Part model, mm, in its own coordinate system. A direction names the side the tool comes from. Give positions to 0.01 mm unless a question says otherwise; leave off trailing zeros. Write each loop counter-clockwise with the first axis right and the second up, starting at its lowest first coordinate (ties: lowest second). Pieces come first, ordered by that corner, then holes. Notation, with made-up numbers: (4.5, 77) - (18.5, 77) arc R26 cw to (18.5, 103) - close; hole circle Ø6 at (61, 10). An arc over 180 degrees is marked (long way). Answer in a Markdown table with one row per item. Add a question column.
1. Band-saw the part on B-B on y = -3. Write the cut outline in (x, z), plus the area to 3 significant figures.
2. Drop flat-ended pins along their axis: pin 1 Ø1.5 at (x, z) = (11, -72) entering from -Y; pin 2 Ø4.5 at (x, z) = (1, -8) entering from +Y; pin 3 Ø12 at (y, z) = (9, -81.5) entering from +X. Give the stop position or say it passes through.
3. Probe line 1 along Z through (x, y) = (8, -3.5); line 2 along Z through (x, y) = (-10, -13); line 3 along Y through (x, z) = (-1, -3). List the from-to ranges inside material, lowest first.
4. Band-saw the part on D-D on y = -10. Write the cut outline in (x, z), plus the area to 3 significant figures.
5. Which spindle directions (+Z, -Z, +X, -X, +Y, -Y) get a long thin tool onto all of the face, cutting with end or side? Do faces 1 (the flat face through (4.03, -2.29, 12.08)), 2 (the flat face through (1, 5, -31.75)), 3 (the flat face through (-4.03, 2.29, 12.08)). Say none if no direction does.
Autodesk Inventor part; units mm, degrees
ref_plane "YZ Plane" through (0, 0, 0) normal (1, 0, 0) x (0, 1, 0)
ref_plane "XZ Plane" through (0, 0, 0) normal (0, 1, 0) x (-1, 0, 0)
ref_plane "XY Plane" through (0, 0, 0) normal (0, 0, 1) x (1, 0, 0)
sketch "Sketch1" plane through (0, 0, 0) normal (0, 0, 1) x (1, 0, 0)
  line L0 (5.4993, 0) -> (2.7496, -4.7625)
  line L1 (2.7496, -4.7625) -> (-2.7496, -4.7625)
  line L2 (-2.7496, -4.7625) -> (-5.4993, 0)
  line L3 (-5.4993, 0) -> (-2.7496, 4.7625)
  line L4 (-2.7496, 4.7625) -> (2.7496, 4.7625)
  line L5 (2.7496, 4.7625) -> (5.4993, 0)
  circle A0 centre (0, 0) radius 0.0127
  dimension "d0" = 9.525
  dimension "d6" = 0.0254
extrude "Extrusion2" add sketch "Sketch1" along normal mid plane 114.3
sketch "Sketch4" plane through (0, 0, -57.15) normal (0, 0, -1) x (-1, 0, 0)
  circle A0 centre (0, 0) radius 0.0127
  circle A1 centre (0, 0) radius 12.7
  dimension "d10" = 25.4
extrude "Extrusion4" add sketch "Sketch4" against normal blind 19.05
thicken "Reduce Hex Shaft" operation add thickness 0.127 both sides no extend neighbours yes toward (0, -1, 0) faces at (0.9165, 4.7625, -6.35) (4.5827, 1.5875, -6.35) (3.6662, -3.175, -6.35) (-3.6662, 3.175, -6.35) (-4.5827, -1.5875, -6.35) (-0.9165, -4.7625, -6.35)
sketch "Sketch5" plane through (0, 0, -38.1) normal (0, 0, 1) x (1, 0, 0)
  circle A0 centre (0, 0) radius 6.35
  dimension "d15" = 12.7
extrude "Extrusion5" add sketch "Sketch5" along normal blind 6.35
thicken "Reduce Base Bushing" operation add thickness 0.127 both sides no extend neighbours yes toward (-0.9967573, 0.0804666, 0) faces at (6.3294, -0.511, -33.8667)
sketch "Sketch8" plane through (0, 0, -57.15) normal (0, 0, -1) x (-1, 0, 0)
  circle A0 centre (0, 0) radius 19.05
  dimension "d28" = 38.1
extrude "Extrusion7" add sketch "Sketch8" along normal blind 50.8
equation "\"d0\" = hexSize"
equation "\"d4\" = length"
equation "\"d13\" = printOffset"
equation "\"d14\" = printOffset"
equation "\"d15\" = bushingForBaseHole"
equation "\"d16\" = sideOfBase"
equation "\"d20\" = printOffset"
equation "\"d21\" = printOffset"
equation "\"hexSize\" = 9.525"
equation "\"length\" = 114.3"
equation "\"printOffset\" = 0.127"
equation "\"bushingForBaseHole\" = 12.7"
equation "\"sideOfBase\" = 6.35"
properties part number "3_8x6_5-inchHexShaft" material "PC/ABS Plastic"
Values:
| question | item | result |
|---|---|---|
| 1 | outline | (-18.81, -107.95) - (18.81, -107.95) - (18.81, -57.15) - (12.34, -57.15) - (12.34, -38.1) - (5.45, -38.1) - (5.45, -31.75) - (3.62, -31.75) - (3.62, 57.15) - (-3.62, 57.15) - (-3.62, -31.75) - (-5.45, -31.75) - (-5.45, -38.1) - (-12.34, -38.1) - (-12.34, -57.15) - (-18.81, -57.15) - close |
| 1 | area | 3,090 mm² |
| 2 | pin 1 | stops at y = -16.06 |
| 2 | pin 2 | stops at y = 4.64 |
| 2 | pin 3 | stops at x = 18.81 |
| 3 | line 1 | z = -107.95 to -38.1 |
| 3 | line 2 | z = -107.95 to -57.15 |
| 3 | line 3 | y = -4.64 to 4.64 |
| 4 | outline | (-16.21, -107.95) - (16.21, -107.95) - (16.21, -57.15) - (7.83, -57.15) - (7.83, -38.1) - (-7.83, -38.1) - (-7.83, -57.15) - (-16.21, -57.15) - close |
| 4 | area | 1,950 mm² |
| 5 | face 1 | +Z, +X, -Y |
| 5 | face 2 | +Z |
| 5 | face 3 | +Z, -X, +Y |
